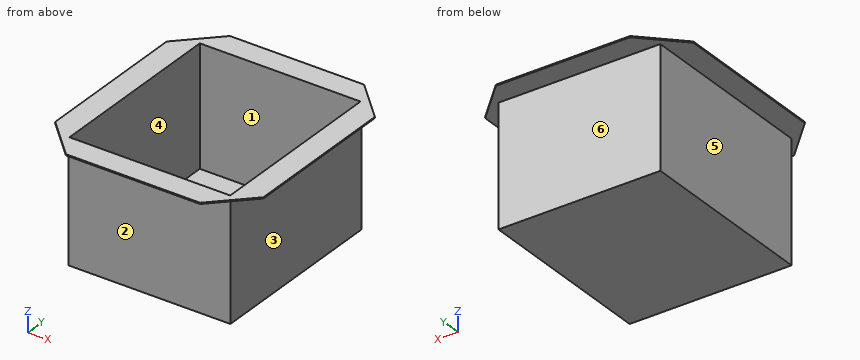
from build123d import *

# Parameters (mm, degrees)
F0_W     = 175
F0_H     = 200
F1_DEPTH = 130
F2_W     = 225
F2_H     = 250
F3_DEPTH = 1.3
F4_W     = 173.7
F4_H     = 198.7
F5_DEPTH = 128.7
F6_SIZE  = 40


with BuildPart() as f1:
    # F0 (on Top) → F1 (new body)
    with BuildSketch(Plane.XY):
        Rectangle(F0_W, F0_H)
    extrude(amount=F1_DEPTH)

    # F2 (on face) → F3 (join)
    with BuildSketch(Plane.XY.offset(130)):
        Rectangle(F2_W, F2_H)
    extrude(amount=F3_DEPTH)

    # F4 (on face) → F5 (cut)
    with BuildSketch(Plane.XY.offset(131.3)):
        Rectangle(F4_W, F4_H)
    extrude(amount=-F5_DEPTH, mode=Mode.SUBTRACT)

    # F6
    f6_edges = [f1.edges().sort_by_distance(p)[0] for p in [
        (112.5, -125, 130.65),
        (-112.5, -125, 130.65),
        (112.5, 125, 130.65),
        (-112.5, 125, 130.65),
    ]]
    chamfer(f6_edges, length=F6_SIZE)


solid = f1.part
Input: part model. Units: mm. Frame: model coordinates. Face numbers are marked on the shaded views. A direction names the side the tool comes from. Give positions to 0.01 mm unless a question says otherwise; leave off trailing zeros. Order: outer loops, then holes, each group sorted by start corner. A loop starts at its lowest first (then second) coordinate and runs counter-clockwise, first axis right, second up. Notation, with made-up numbers: M 2.5,56 L 14.5,56 A16 cw 14.5,60 Z; hole C 64.5,50 d7. An arc over 180 degrees is marked long. Answer as a JSON object with one key per item and string values.
1. Cut plane C-C, the plane x = 82. Output: boundary loops of the cut face in (y, z).
Result sheet:
{"outline": "M -115.5,130 L -100,130 L -100,0 L 100,0 L 100,130 L 115.5,130 L 115.5,131.3 L 99.35,131.3 L 99.35,2.6 L -99.35,2.6 L -99.35,131.3 L -115.5,131.3 Z"}
2. Cut plane B-B, the plane y = 39. Output: boundary loops of the cut face in (x, z).
Result sheet:
{"outline": "M -112.5,130 L -87.5,130 L -87.5,0 L 87.5,0 L 87.5,130 L 112.5,130 L 112.5,131.3 L 86.85,131.3 L 86.85,2.6 L -86.85,2.6 L -86.85,131.3 L -112.5,131.3 Z"}
3. Pull-direction query (Y, two-part tool) for the marked faces 1, 2 and 3; classes: +Y half, -Y half, draft (parallel to the pull), parting line (faces both ways), or undercut.
Result sheet:
{"face 1": "undercut", "face 2": "-Y half", "face 3": "draft"}
4. Ray query, line 1 (X direction, y = 11, z = 40); line 2 (Y direction, x = -50, z = 14); line 3 (Z direction, x = 63.5, y = -17). Return the intervals inside material, ascending. Write a range as [from, to].
Result sheet:
{"line 1": "[-87.5, -86.85], [86.85, 87.5]", "line 2": "[-100, -99.35], [99.35, 100]", "line 3": "[0, 2.6]"}
5. First-contact query: P1, Ø5, axis at x = 42, y = -15, coming from the +Z side; P2, Ø5, axis at x = -18.5, z = 24, coming from the +Y side; P3, Ø1.5, axis at y = 68.5, z = 98, coming from the -X side. Flat tips, straight axial feed; report the tip coordinate or a pass-through.
Result sheet:
{"P1": "z = 2.6", "P2": "y = 100", "P3": "x = -87.5"}
6. Reachability of the marked faces 4, 5 and 6 from +Z, -Z, +X, -X, +Y, -Y: full face, straight path, thin tool, end or side. Return the list, or none.
Result sheet:
{"face 4": "+Z", "face 5": "-Z, -X, +Y, -Y", "face 6": "-Z, +X, -X, +Y"}
7. Cut plane A-A, the plane z = 45. Output: boundary loops of the cut face in (x, y).
Result sheet:
{"outline": "M -87.5,-100 L 87.5,-100 L 87.5,100 L -87.5,100 Z; hole M -86.85,-99.35 L 86.85,-99.35 L 86.85,99.35 L -86.85,99.35 Z"}
